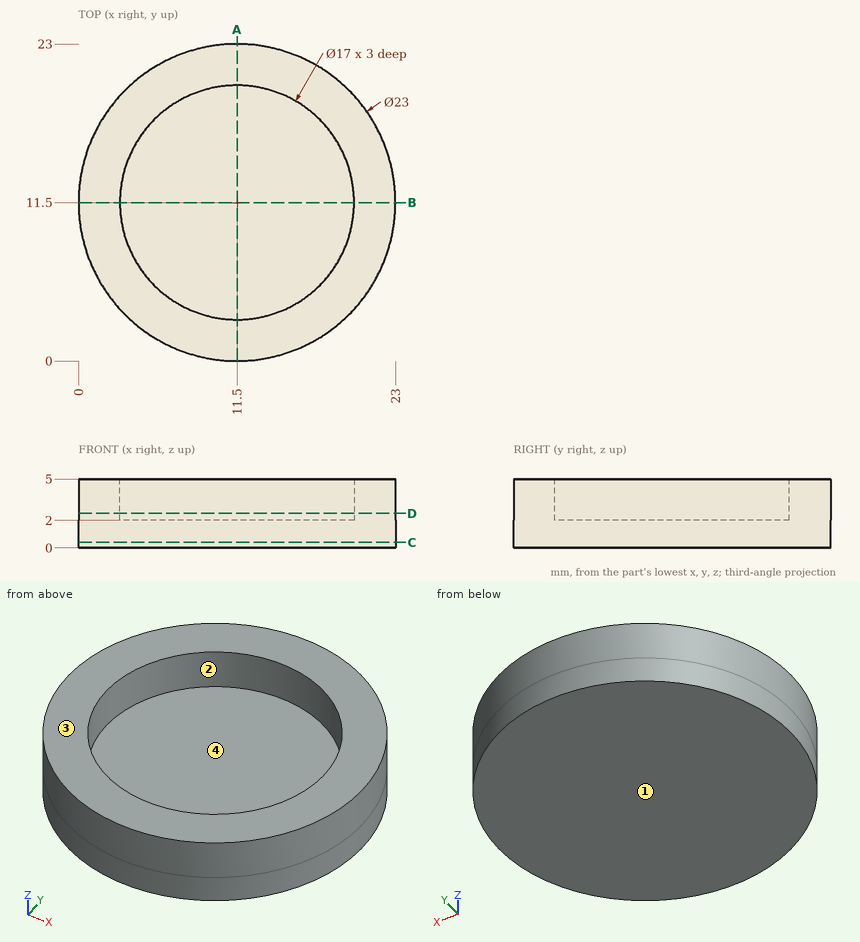
Part print with two shaded views. Sizes in mm from the minimum x, y, z corner. A direction names the side the tool comes from. Coordinates: 2 decimals unless noted, no trailing zeros. Write each loop counter-clockwise with the first axis right and the second up, starting at its lowest first coordinate (ties: lowest second). Pieces come first, ordered by that corner, then holes.
1. Drop flat-ended pins along their axis: pin 1 (1.5 mm diameter, centred on y = 5, z = 3.5, fed in from +X); pin 2 (1.5 mm diameter, centred on x = 6, z = 2, fed in from +Y); pin 3 (2 mm diameter, centred on x = 19.5, z = 0.5, fed in from -Y). Give the stop position or say it passes through.
Answer block:
pin 1: stops at x = 21.46
pin 2: stops at y = 21.97
pin 3: stops at y = 2.38
2. Band-saw the part on C-C, the plane z = 0.4. Give the cut face in (x, y).
Answer block:
outline: circle Ø23 at (11.5, 11.5)
3. Band-saw the part on A-A, the plane x = 11.5. Give the cut face in (y, z), and give its area (3 significant figures).
Answer block:
outline: (0, 0) - (23, 0) - (23, 5) - (20, 5) - (20, 2) - (3, 2) - (3, 5) - (0, 5) - close
area: 64.0 mm2
4. Drill centre lines: probe 1 along Y at (x, z) = (11.5, 4); probe 2 along Z at (x, y) = (15.5, 11.75); probe 3 along Y at (x, z) = (7, 2.95). Where is each one in solid material? Low to high.
Answer block:
probe 1: y = 0 to 3, 20 to 23
probe 2: z = 0 to 2
probe 3: y = 0.92 to 4.29, 18.71 to 22.08
5. 3-axis set-ups, long thin cutter, end or side, ignore diameter. For the marked faces 3 and 4: which of +Z, -Z, +X, -X, +Y, -Y reach the whole face in a straight line?
Answer block:
face 3: +Z, +X, -X, +Y, -Y
face 4: +Z
6. Band-saw the part on D-D, the plane z = 2.5. Give the cut face in (x, y), and give its area (3 significant figures).
Answer block:
outline: circle Ø23 at (11.5, 11.5); hole circle Ø17 at (11.5, 11.5)
area: 188 mm2
7. Pull direction X, two halves, no side cores. Call the marked faces 1 and 2: released by +X, released by -X, zero draft, split by the parting line, or undercut.
Answer block:
face 1: zero draft
face 2: undercut
